Could you check a few things on this drawing? It's one solid part, dimensions in mm from its lowest x, y, z. A direction names the side the tool comes from. Round coordinates to 2 decimals unless told otherwise and drop trailing zeros. Loops run counter-clockwise (first coordinate to the right, second up) from the corner with the lowest first, then second, coordinate; pieces in that order, holes last. Notation, with made-up numbers: M 79,40.5 L 136,40.5 A35 cw 136,73.5 Z; hole C -4,57 d9. An arc over 180 degrees is marked long. Return JSON: item names as keys, results as strings.
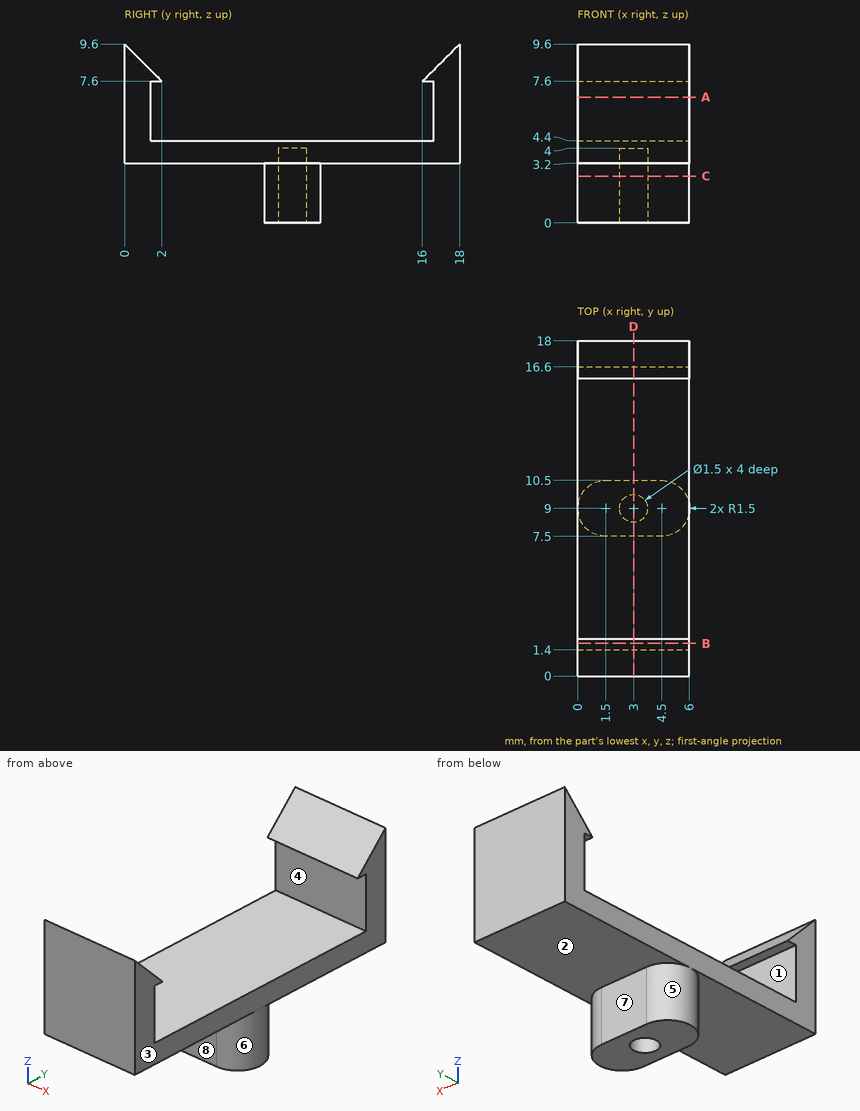
Q1. Thinking about a two-plate mould opening in Z: for the marked faces 1, 2 and 3, which applies, pulls with the +Z half, pulls with the -Z half, needs draft (parallel to the pull), parting line crosses it, or undercut?
Results:
{"face 1": "undercut", "face 2": "pulls with the -Z half", "face 3": "needs draft"}
Q2. Suppose I cut it at A-A, the plane z = 6.75. Please give me the cut outline in (x, y), plus the area to 3 significant figures.
Results:
{"outline": "M 0,0 L 6,0 L 6,1.4 L 0,1.4 Z; M 0,16.6 L 6,16.6 L 6,18 L 0,18 Z", "area": "16.8 mm2"}
Q3. Suppose I cut it at D-D, the plane x = 3. Please give me the cut outline in (y, z).
Results:
{"outline": "M 0,3.2 L 7.5,3.2 L 7.5,0 L 8.25,0 L 8.25,4 L 9.75,4 L 9.75,0 L 10.5,0 L 10.5,3.2 L 18,3.2 L 18,9.6 L 16,7.6 L 16.6,7.6 L 16.6,4.4 L 1.4,4.4 L 1.4,7.6 L 2,7.6 L 0,9.6 Z"}
Q4. On a 3-axis mill with a long thin cutter (end or side, diameter ignored), from which of +Z, -Z, +X, -X, +Y, -Y can I reach the whole of each face in a straight line? I mean the marked faces 4, 5, 6, 7 and 8. Say none if no direction works.
Results:
{"face 4": "+X, -X", "face 5": "-Z, -X", "face 6": "-Z, +X", "face 7": "-Z, +X, -X, +Y", "face 8": "-Z, +X, -X, -Y"}
Q5. Suppose I cut it at B-B, the plane y = 1.75. Please give me the cut outline in (x, z), plus the area to 3 significant figures.
Results:
{"outline": "M 0,3.2 L 6,3.2 L 6,4.4 L 0,4.4 Z; M 0,7.6 L 6,7.6 L 6,7.85 L 0,7.85 Z", "area": "8.70 mm2"}
Q6. If I drill on line 1 along Y through (x, z) = (3, 2.05); line 2 along Y through (x, z) = (2.85, 6.75); line 3 along Z through (x, y) = (3.1, 3.75), over which ranges is the centre line in solid material (lowest first)?
Results:
{"line 1": "y = 7.5 to 8.25, 9.75 to 10.5", "line 2": "y = 0 to 1.4, 16.6 to 18", "line 3": "z = 3.2 to 4.4"}
Q7. I'm going to push flat-ended pins straight in: pin 1 Ø2.5 at (x, y) = (3, 9) entering from -Z; pin 2 Ø3 at (x, z) = (4.5, 1.5) entering from +Y; pin 3 Ø0.5 at (x, y) = (4, 2) entering from -Z; pin 4 Ø1.8 at (x, y) = (2.5, 5.5) entering from +Z. Where does each tip first touch, or does it pass through?
Results:
{"pin 1": "stops at z = 0", "pin 2": "stops at y = 10.5", "pin 3": "stops at z = 3.2", "pin 4": "stops at z = 4.4"}
Q8. Suppose I cut it at C-C, the plane z = 2.5. Please give me the cut outline in (x, y), plus the area to 3 significant figures.
Results:
{"outline": "M 1.5,7.5 L 4.5,7.5 A1.5 ccw 4.5,10.5 L 1.5,10.5 A1.5 ccw Z; hole C 3,9 d1.5", "area": "14.3 mm2"}
